Could you check a few things on this model? Use its own coordinates, in mm. A direction names the side the tool comes from. Give positions to 0.01 mm unless a question says otherwise; leave off trailing zeros. Order: outer loops, then holes, each group sorted by start corner. A loop starts at its lowest first (then second) coordinate and runs counter-clockwise, first axis right, second up. Notation, with made-up numbers: (38, 40.5) -> (46, 40.5) arc R23 cw to (46, 56.5) -> close; hole circle Ø9 at (18, 33). An arc over 180 degrees is marked (long way). One line per item, written item: value.
Autodesk Inventor part; units mm, degrees
ref_plane "YZ Plane" through (0, 0, 0) normal (1, 0, 0) x (0, 1, 0)
ref_plane "XZ Plane" through (0, 0, 0) normal (0, 1, 0) x (-1, 0, 0)
ref_plane "XY Plane" through (0, 0, 0) normal (0, 0, 1) x (1, 0, 0)
sketch "Sketch1" plane through (0, 0, 0) normal (0, 1, 0) x (-1, 0, 0)
  circle A0 centre (25.5, 34.24) radius 1.75
  circle A1 centre (-25.5, 34.24) radius 1.75
  line L0 (23.7877, 30) -> (26.625, 30)
  arc A2 (21.7877, 32) -> (23.7877, 30) centre (23.7877, 32) ccw
  line L1 (21.7877, 35.55) -> (21.7877, 32)
  arc A3 (21.7877, 35.55) -> (21.7387, 35.99) centre (19.7877, 35.55) ccw
  arc A4 (28.625, 28) -> (26.625, 30) centre (26.625, 28) ccw
  line L2 (-21.7877, 32) -> (-21.7877, 35.55)
  arc A5 (-21.7387, 35.99) -> (-21.7877, 35.55) centre (-19.7877, 35.55) ccw
  arc A6 (-23.7877, 30) -> (-21.7877, 32) centre (-23.7877, 32) ccw
  line L3 (-26.625, 30) -> (-23.7877, 30)
  arc A7 (-26.625, 30) -> (-28.625, 28) centre (-26.625, 28) ccw
  line L4 (28.625, 28) -> (28.625, 35.99)
  line L5 (-28.625, 28) -> (-28.625, 35.99)
  line L6 (21.7877, 34.24) -> (-21.7877, 34.24)
  line L7 (28.625, 35.99) -> (-28.625, 35.99)
  line L8 (21.7877, 32) -> (-21.7877, 32)
  line L9 (-28.625, 35.99) -> (28.625, 35.99)
  line L10 (28.625, 35.99) -> (28.625, 37.99)
  line L11 (28.625, 37.99) -> (-28.625, 37.99)
  line L12 (-28.625, 37.99) -> (-28.625, 35.99)
  dimension "d6" = 2
extrude "Extrusion1" add sketch "Sketch1" along normal blind 2 contours L7 L4 A4 L0 A2 L1 A3 | A5 L2 A6 L3 A7 L5 L7
extrude "Extrusion2" add sketch "Sketch1" along normal blind 15 contours A3 L1 L6 L2 A5 L7
extrude "Extrusion3" add sketch "Sketch1" along normal blind 1 contours L1 L8 L2 L6
extrude "Extrusion4" add sketch "Sketch1" along normal blind 2 contours L7 L12 L11 L10
properties part number "pelindung uvtron"
1) Suppose I cut it at A-A, the plane x = -25.5. Write out the boundary of the cut face in (y, z), then the cut area to 3 significant figures.
Answer below:
outline: (0, 30) -> (2, 30) -> (2, 32.49) -> (0, 32.49) -> close; (0, 35.99) -> (2, 35.99) -> (2, 37.99) -> (0, 37.99) -> close
area: 8.98 mm2
2) Suppose I cut it at B-B, the plane z = 31.25. Write out the boundary of the cut face in (x, y) (3 decimals).
Answer below:
outline: (-28.625, 0) -> (-21.934, 0) -> (-21.934, 2) -> (-28.625, 2) -> close; (21.934, 0) -> (28.625, 0) -> (28.625, 2) -> (21.934, 2) -> close
3) For faces 1 (the flat face through (0, 1, 33)), 2 (the flat face through (-21.788, 8, 35)), 3 (the cylindrical face through (22.36, 0.99, 30.6)), 4 (the flat face through (0, 8, 35.99)), which set-ups out of +Z, -Z, +X, -X, +Y, -Y let a thin tool reach every point of the face, with its end or its side?
Answer below:
face 1: -Z, +Y
face 2: +Z, -Z, -X, +Y
face 3: -Z, +Y, -Y
face 4: +Z, +X, -X, +Y
4) We'd pull the mould along Z, two halves only. Please class faces 5 (the cylindrical face through (-23.75, 0.99, 34.16)), 6 (the flat face through (25, 1, 30)), 7 (the flat face through (0, 0, 35)): +Z half, -Z half, draft (parallel to the pull), parting line (faces both ways), or undercut.
Answer below:
face 5: undercut
face 6: -Z half
face 7: draft
5) Suppose I cut it at D-D, the plane x = 18.5. Write out the boundary of the cut face in (y, z).
Answer below:
outline: (0, 32) -> (1, 32) -> (1, 34.24) -> (15, 34.24) -> (15, 35.99) -> (2, 35.99) -> (2, 37.99) -> (0, 37.99) -> close
6) Suppose I cut it at C-C, the plane y = 2.5. Write out the boundary of the cut face in (x, z).
Answer below:
outline: (-21.79, 34.24) -> (21.79, 34.24) -> (21.79, 35.55) arc R2 ccw to (21.74, 35.99) -> (-21.74, 35.99) arc R2 ccw to (-21.79, 35.55) -> close
7) If I drill on line 1 along Z through (x, y) = (25.5, 0.85); line 2 along Y through (x, z) = (-20, 36.5); line 3 along Y through (x, z) = (1.5, 34), over which ranges is the centre line in solid material (lowest first)?
Answer below:
line 1: z = 30 to 32.49, 35.99 to 37.99
line 2: y = 0 to 2
line 3: y = 0 to 1
8) For P1, Ø4, axis at x = -3.5, z = 29.5, coming from the -Y side; P2, Ø6.5, axis at x = 3, y = 7, coming from the +Z side; P3, Ø1, axis at x = -26, y = 1, coming from the -Z side; P4, Ø1, axis at y = 11, z = 35, coming from the +X side, each with a flat end and sliding along its axis, tell me the tip position at first contact or that it passes through.
Answer below:
P1: passes through
P2: stops at z = 35.99
P3: stops at z = 30
P4: stops at x = 21.79
